Read the model definition and answer for the solid it produces. Units are mm, in the model's axes. A direction names the side the tool comes from. Give positions to 0.01 mm unless a question says otherwise; leave off trailing zeros. Loops run counter-clockwise (first coordinate to the right, second up) from the corner with the lowest first, then second, coordinate; pieces in that order, holes last. Notation, with made-up numbers: (27, 1) - (66, 1) arc R22 ccw to (66, 29) - close; hole circle Ø7 at (83.25, 65). An arc over 180 degrees is marked (long way). Write each question's results on one line, items separated by ' | '. Start each with the question number.
Q1. Given pin 1 (0.8 mm diameter, centred on x = -26, z = 1.5, fed in from +Y); pin 2 (6 mm diameter, centred on x = -13.5, z = 6.5, fed in from -Y); pin 3 (0.9 mm diameter, centred on x = -2, z = 12, fed in from -Y); pin 4 (6.5 mm diameter, centred on x = 3, y = -51.5, fed in from +Z), each flat-ended and moving along its own axis, determine where each tip first touches the part or whether it passes through.
Q2. Determine the mould class of faces 4 (the cylindrical face through (23.762, -45.756, 1.503)), 5 (the flat face through (27, -44.082, 2)), 6 (the cylindrical face through (17.648, 54.347, 12.425)), 7 (the flat face through (-27.94, -23, 2)) for opening direction X: +X half, -X half, draft (parallel to the pull), parting line (faces both ways), or undercut.
Q3. For faces 1 (the flat face through (27, 1.638, 2)), 2 (the cylindrical face through (-19.594, -54.731, 12.425)), 3 (the flat face through (22.098, -1, 8)), determine the directions among +Z, -Z, +X, -X, +Y, -Y from which every point of the face is accessible in a straight line to the end or side of a thin tool.
Q4. The part is cut by section A-A, the plane y = -39.5. Write down the section's boundary in (x, z), plus the area to 3 significant figures.
Q5. Find the intervals of material crossed by line 1 (Y direction, x = -12, z = 12); line 2 (X direction, y = -18.5, z = 3.5); line 3 (Z direction, x = -4.5, y = 44), in increasing order. Write a range as from..to.
Q6. The part is cut by section B-B, the plane z = 6.5. Write down the section's boundary in (x, y), plus the area to 3 significant figures.
```python
from build123d import *

# Parameters (mm, degrees)
F1_DEPTH  = 3.048
F2_SIZE   = 3.81
F3_R      = 1.524
F4_W      = 44.196
F4_H      = 114.3
F5_DEPTH  = 9.652
F6_W      = 44.196
F6_H      = 12.7
F7_DEPTH  = 1.778
F8_R      = 2.286
F9_DEPTH  = 3.048
F10_R     = 1.016
F11_DEPTH = 3.048


with BuildPart() as f1:
    # F0 (on Top) → F1 (new body)
    with BuildSketch(Plane.XY):
        with BuildLine():
            Line((-27.94, -58.42), (27.94, -58.42))
            Line((27.94, -58.42), (27.94, -47.3583))
            Line((27.94, -47.3583), (25.4, -47.3583))
            ThreePointArc((25.4, -47.3583), (23.7617, -45.72), (25.4, -44.0817))
            Line((25.4, -44.0817), (27.94, -44.0817))
            Line((27.94, -44.0817), (27.94, -1.6383))
            Line((27.94, -1.6383), (25.4, -1.6383))
            ThreePointArc((25.4, -1.6383), (23.7617, 0), (25.4, 1.6383))
            Line((25.4, 1.6383), (27.94, 1.6383))
            Line((27.94, 1.6383), (27.94, 44.0817))
            Line((27.94, 44.0817), (25.4, 44.0817))
            ThreePointArc((25.4, 44.0817), (23.7617, 45.72), (25.4, 47.3583))
            Line((25.4, 47.3583), (27.94, 47.3583))
            Line((27.94, 47.3583), (27.94, 58.42))
            Line((27.94, 58.42), (-27.94, 58.42))
            Line((-27.94, 58.42), (-27.94, 47.3583))
            Line((-27.94, 47.3583), (-25.4, 47.3583))
            ThreePointArc((-25.4, 47.3583), (-24.241547, 46.878453), (-23.7617, 45.72))
            ThreePointArc((-23.7617, 45.72), (-24.241547, 44.561547), (-25.4, 44.0817))
            Line((-25.4, 44.0817), (-27.94, 44.0817))
            Line((-27.94, 44.0817), (-27.94, 1.6383))
            Line((-27.94, 1.6383), (-25.4, 1.6383))
            ThreePointArc((-25.4, 1.6383), (-24.241547, 1.158453), (-23.7617, 0))
            ThreePointArc((-23.7617, 0), (-24.241547, -1.158453), (-25.4, -1.6383))
            Line((-25.4, -1.6383), (-27.94, -1.6383))
            Line((-27.94, -1.6383), (-27.94, -44.0817))
            Line((-27.94, -44.0817), (-25.4, -44.0817))
            ThreePointArc((-25.4, -44.0817), (-24.241547, -44.561547), (-23.7617, -45.72))
            ThreePointArc((-23.7617, -45.72), (-24.241547, -46.878453), (-25.4, -47.3583))
            Line((-25.4, -47.3583), (-27.94, -47.3583))
            Line((-27.94, -47.3583), (-27.94, -58.42))
        make_face()
    extrude(amount=F1_DEPTH)

    # F2
    f2_edges = [f1.edges().sort_by_distance(p)[0] for p in [
        (-27.94, 58.42, 1.524),
    ]]
    chamfer(f2_edges, length=F2_SIZE)

    # F3
    f3_edges = [f1.edges().sort_by_distance(p)[0] for p in [
        (27.94, 58.42, 1.524),
        (27.94, -58.42, 1.524),
        (-27.94, -58.42, 1.524),
    ]]
    fillet(f3_edges, radius=F3_R)

    # F4 (on face) → F5 (join)
    with BuildSketch(Plane.XY.offset(3.048)):
        Rectangle(F4_W, F4_H)
    extrude(amount=F5_DEPTH)

    # F6 (on face) → F7 (cut)
    with BuildSketch(Plane.XY.offset(12.7)):
        with Locations((0, -50.8)):
            Rectangle(F6_W, F6_H)
        with Locations((0, 50.8)):
            Rectangle(F6_W, F6_H)
    extrude(amount=-F7_DEPTH, mode=Mode.SUBTRACT)

    # F8 (on face) → F9 (join)
    with BuildSketch(Plane.XY.offset(10.922)):
        with Locations((-17.78, -53.34)):
            Circle(F8_R)
        with Locations((17.78, -53.34)):
            Circle(F8_R)
    extrude(amount=F9_DEPTH)

    # F10 (on face) → F11 (join, through all)
    with BuildSketch(Plane.XY.offset(10.922)):
        with Locations((-7.62, -53.34)):
            Circle(F10_R)
        with Locations((0, -53.34)):
            Circle(F10_R)
        with Locations((7.62, -53.34)):
            Circle(F10_R)
        with Locations((-17.78, 53.34)):
            Circle(F10_R)
        with Locations((-7.62, 53.34)):
            Circle(F10_R)
        with Locations((7.62, 53.34)):
            Circle(F10_R)
        with Locations((17.78, 53.34)):
            Circle(F10_R)
    extrude(amount=F11_DEPTH)


solid = f1.part
```
Check sheet entries:
1) pin 1: stops at y = 56.95 | pin 2: stops at y = -57.15 | pin 3: stops at y = -44.45 | pin 4: stops at z = 13.97
2) face 4: +X half | face 5: draft | face 6: undercut | face 7: -X half
3) face 1: +Z, -Z, +X | face 2: +Z | face 3: +Z, +X, +Y, -Y
4) outline: (-27.94, 0) - (27.94, 0) - (27.94, 3.05) - (22.1, 3.05) - (22.1, 12.7) - (-22.1, 12.7) - (-22.1, 3.05) - (-27.94, 3.05) - close | area: 597 mm^2
5) line 1: y = -44.45..44.45 | line 2: x = -22.1..22.1 | line 3: z = 0..12.7
6) outline: (-22.1, -57.15) - (22.1, -57.15) - (22.1, 57.15) - (-22.1, 57.15) - close | area: 5,050 mm^2
